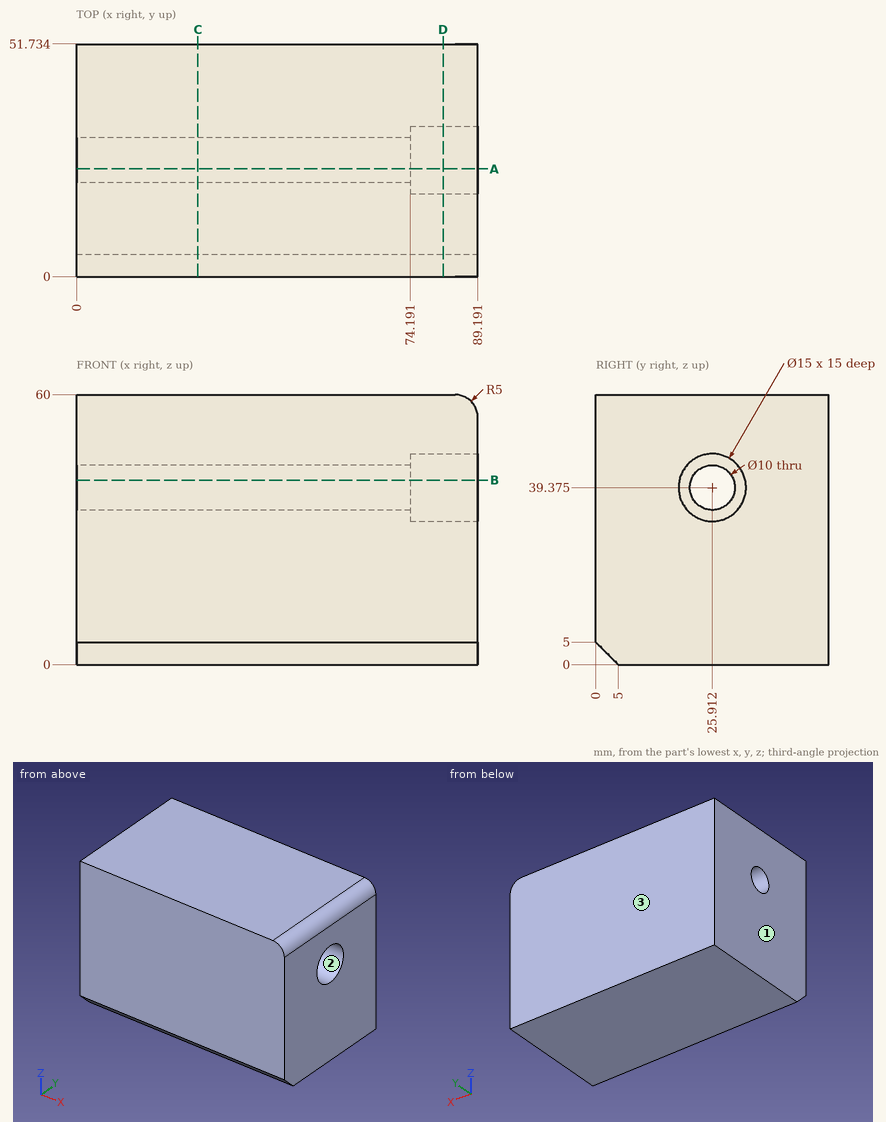
Input: dimensioned drawing with shaded views. Units: mm. Origin: part minimum x, y, z. Give positions to 0.01 mm unless a question says otherwise; leave off trailing zeros. Write each loop counter-clockwise with the first axis right and the second up, starting at its lowest first coordinate (ties: lowest second). Pieces come first, ordered by that corner, then holes. Notation, with made-up numbers: (7.25, -2) -> (50.25, -2) arc R16 ccw to (50.25, 2) -> close; hole circle Ø7 at (-19, 29.5). An arc over 180 degrees is marked (long way). Return JSON: item names as keys, results as strings. Group by question number.
1. Section D-D, the plane x = 81.5. Output: boundary loops of the cut face in (y, z) (1 decimal).
2. Material intervals for line 1 (Z direction, x = 6.5, y = 26); line 2 (Z direction, x = 43.5, y = 29); line 3 (Y direction, x = 53.5, z = 36) (1 decimal), sorted ascending. Write a range as from..to.
3. Section A-A, the plane y = 24. Output: boundary loops of the cut face in (x, z) (1 decimal).
4. Mould query, pull axis Y, two halves, no side actions, for the marked faces 1, 2 and 3. Classes: +Y half, -Y half, draft (parallel to the pull), parting line (faces both ways), or undercut.
5. Section B-B, the plane z = 41. Output: boundary loops of the cut face in (x, y), then the cut area to 3 significant figures.
6. Section C-C, the plane x = 27. Output: boundary loops of the cut face in (y, z) (1 decimal), then the cut area to 3 significant figures.
Determined:
{
 "1": {"outline": "(0, 5) -> (5, 0) -> (51.7, 0) -> (51.7, 60) -> (0, 60) -> close; hole circle Ø15 at (25.9, 39.4)"},
 "2": {"line 1": "z = 0..34.38, 44.37..60", "line 2": "z = 0..35.44, 43.31..60", "line 3": "y = 0..22.2, 29.6..51.7"},
 "3": {"outline": "(0, 0) -> (89.2, 0) -> (89.2, 32.1) -> (74.2, 32.1) -> (74.2, 34.8) -> (0, 34.8) -> close; (0, 44) -> (74.2, 44) -> (74.2, 46.6) -> (89.2, 46.6) -> (89.2, 55) arc R5 ccw to (84.2, 60) -> (0, 60) -> close"},
 "4": {"face 1": "draft", "face 2": "undercut", "face 3": "+Y half"},
 "5": {"outline": "(0, 0) -> (89.19, 0) -> (89.19, 18.59) -> (74.19, 18.59) -> (74.19, 21.18) -> (0, 21.18) -> close; (0, 30.64) -> (74.19, 30.64) -> (74.19, 33.23) -> (89.19, 33.23) -> (89.19, 51.73) -> (0, 51.73) -> close", "area": "3,690 mm2"},
 "6": {"outline": "(0, 5) -> (5, 0) -> (51.7, 0) -> (51.7, 60) -> (0, 60) -> close; hole circle Ø10 at (25.9, 39.4)", "area": "3,010 mm2"}
}
